Input: dimensioned drawing with shaded views. Units: mm. Origin: part minimum x, y, z. Round coordinates to 2 decimals unless told otherwise and drop trailing zeros. Order: outer loops, then holes, each group sorted by start corner. A loop starts at its lowest first (then second) coordinate and runs counter-clockwise, first axis right, second up. Notation, with made-up numbers: M 20,-28 L 60,-28 A27 ccw 60,-4 Z; hole C 16.5,49 d6. An arc over 180 degrees is marked long. Answer as CSV lines item,"result". Start each with the question number.
Item 1: Section query C-C on z = 35.5. Return the cut outline in (x, y) (1 decimal), plus the area to 3 significant figures.
Item 2: Section query B-B on z = 20. Return the cut outline in (x, y).
Item 3: Section query A-A on y = 3.95. Return the cut outline in (x, z) (1 decimal).
Item 4: Pull-direction query (Y, two-part tool) for the marked faces 1 and 2; classes: +Y half, -Y half, draft (parallel to the pull), parting line (faces both ways), or undercut.
Item 5: First-contact query: P1, Ø1.5, axis at x = 195.5, y = 2, coming from the +Z side; P2, Ø2.5, axis at y = 2, z = 34.5, coming from the -X side (3 decimals); P3, Ø1, axis at y = 1.5, z = 24, coming from the -X side. Flat tips, straight axial feed; report the tip coordinate or a pass-through.
Item 6: Line query: line 1 (X direction, y = 3.2, z = 20); line 2 (X direction, y = 0.3, z = 21); line 3 (X direction, y = 0.7, z = 38) (1 decimal). Output: solid intervals per line, ascending. Write a range as [from, to].
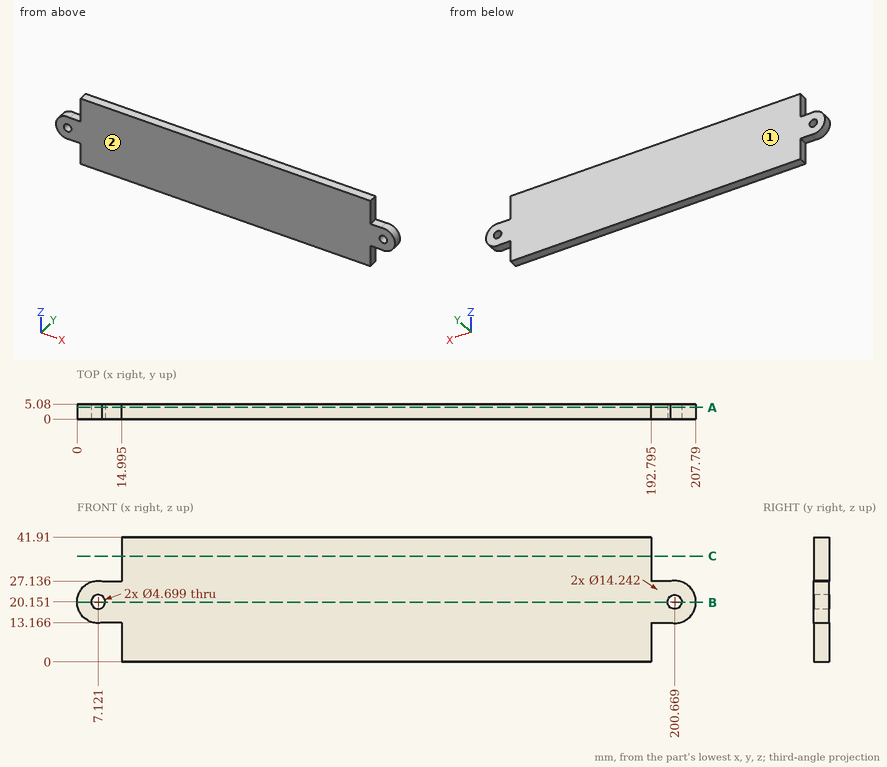
Results:
1,outline,"M 15,0 L 192.8,0 L 192.8,5.1 L 15,5.1 Z"
1,area,"903 mm^2"
2,outline,"M 0,0 L 4.78,0 L 4.78,5.08 L 0,5.08 Z; M 9.47,0 L 198.32,0 L 198.32,5.08 L 9.47,5.08 Z; M 203.01,0 L 207.79,0 L 207.79,5.08 L 203.01,5.08 Z"
3,outline,"M 8.5,13.2 L 15,13.2 L 15,0 L 192.8,0 L 192.8,13.2 L 199.3,13.2 A7.1 ccw long 199.3,27.1 L 192.8,27.1 L 192.8,41.9 L 15,41.9 L 15,27.1 L 8.5,27.1 A7.1 ccw long Z; hole C 7.1,20.2 d4.7; hole C 200.7,20.2 d4.7"
4,face 1,"+Y half"
4,face 2,"-Y half"
5,P1,"z = 27.14"
5,P2,"x = 14.995"
5,P3,"x = 0.84"
6,line 1,"[0, 4.78], [9.47, 198.32], [203.01, 207.79]"
6,line 2,"[0.05, 4.93], [9.31, 198.48], [202.86, 207.74]"
6,line 3,"[15, 192.8]"
